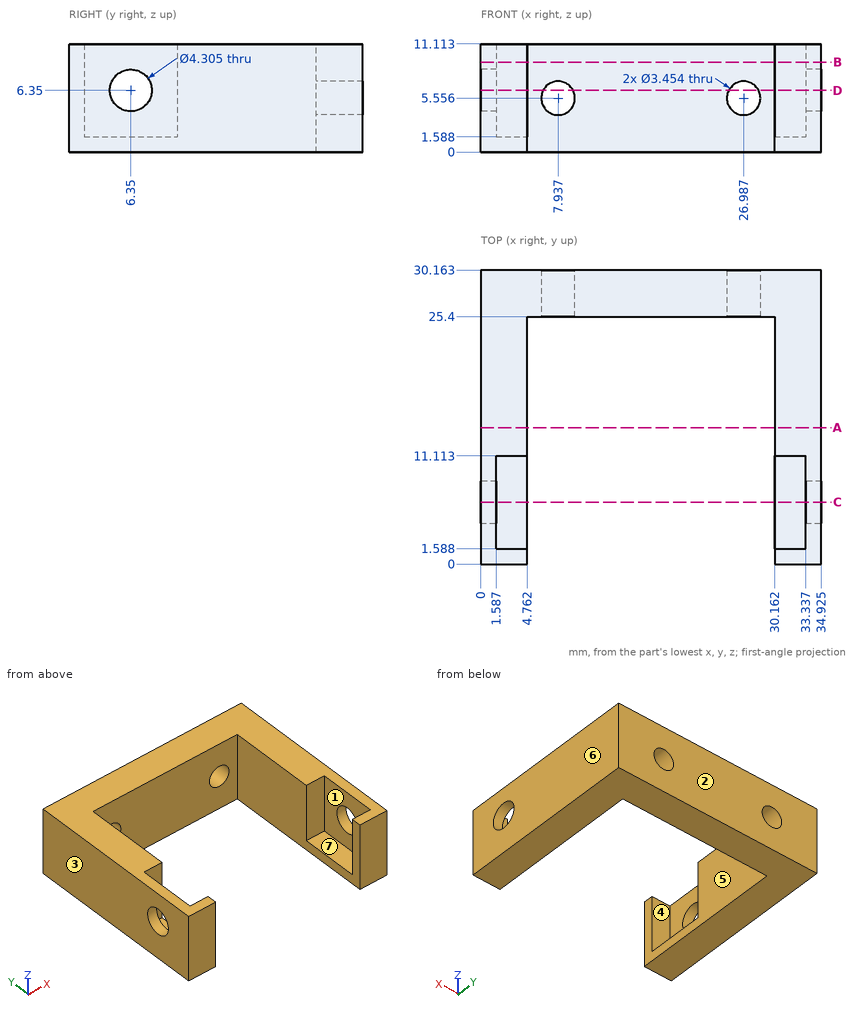
Study the drawing (mm; zero at the part's minimum x, y, z) and answer. A direction names the side the tool comes from. Round coordinates to 2 decimals unless told otherwise and drop trailing zeros. Loops run counter-clockwise (first coordinate to the right, second up) from the corner with the lowest first, then second, coordinate; pieces in that order, holes last.
Q1. Find the intervals of material crossed by line 1 (X direction, y = 3, z = 6.5) (1 decimal); line 2 (Y direction, x = 4, z = 8.25); line 3 (X direction, y = 24, z = 4.5) (1 decimal), in increasing order.
Q2. Given pin 1 Ø1.6 at (x, y) = (3, 6.5) entering from +Z; pin 2 Ø3.5 at (x, z) = (3, 8.5) entering from -Y; pin 3 Ø4 at (x, z) = (17, 7) entering from -Y, each flat-ended and moving along its own axis, determine where each tip first touches the part or whether it passes through.
Q3. Section C-C, the plane y = 6.35 is taken. Determine the outline of the cut face in (x, z) (1 decimal).
Q4. For a pull along Y with two mould halves and no side action, classify the marked faces 1, 2, 3 and 4 as released by +Y, released by -Y, zero draft, split by the parting line, or undercut.
Q5. Section D-D, the plane z = 6.35 is taken. Count the separate pieces of the cut face and the enclosed holes in it, then the cut area to 3 significant figures.
Q6. Section B-B, the plane z = 9.25 is taken. Determine the outline of the cut face in (x, y) (1 decimal).
Q7. Which of the six approach directions +Z, -Z, +X, -X, +Y, -Y give full straight-line access (tool end or side, diameter ignored) to the marked faces 5, 6 and 7?
Q8. Section A-A, the plane y = 14 is taken. Determine the outline of the cut face in (x, z) (1 decimal), then the cut area to 3 significant figures.
Completed:
1. line 1: x = 0 to 1.6, 33.3 to 34.9
1. line 2: y = 0 to 1.59, 11.11 to 30.16
1. line 3: x = 0 to 4.8, 30.2 to 34.9
2. pin 1: stops at z = 1.59
2. pin 2: stops at y = 0
2. pin 3: stops at y = 25.4
3. outline: (0, 0) - (4.8, 0) - (4.8, 1.6) - (1.6, 1.6) - (1.6, 4.2) - (0, 4.2) - close; (0, 8.5) - (1.6, 8.5) - (1.6, 11.1) - (0, 11.1) - close; (30.2, 0) - (34.9, 0) - (34.9, 4.2) - (33.3, 4.2) - (33.3, 1.6) - (30.2, 1.6) - close; (33.3, 8.5) - (34.9, 8.5) - (34.9, 11.1) - (33.3, 11.1) - close
4. face 1: undercut
4. face 2: released by +Y
4. face 3: zero draft
4. face 4: undercut
5. separate pieces: 5
5. enclosed holes: 0
5. area: 305 mm2
6. outline: (0, 0) - (4.8, 0) - (4.8, 1.6) - (1.6, 1.6) - (1.6, 11.1) - (4.8, 11.1) - (4.8, 25.4) - (30.2, 25.4) - (30.2, 11.1) - (33.3, 11.1) - (33.3, 1.6) - (30.2, 1.6) - (30.2, 0) - (34.9, 0) - (34.9, 30.2) - (0, 30.2) - close
7. face 5: +Z, -Z, -Y
7. face 6: +Z, -Z, +X, +Y, -Y
7. face 7: +Z
8. outline: (0, 0) - (4.8, 0) - (4.8, 11.1) - (0, 11.1) - close; (30.2, 0) - (34.9, 0) - (34.9, 11.1) - (30.2, 11.1) - close
8. area: 106 mm2
